Design review of the part shown in the three views and the two pictorial views. Dimensions are in mm from the part's minimum x, y and z. A direction names the side the tool comes from. Give positions to 0.01 mm unless a question says otherwise; leave off trailing zeros. Write each loop counter-clockwise with the first axis right and the second up, starting at its lowest first coordinate (ties: lowest second). Pieces come first, ordered by that corner, then holes. Notation, with made-up numbers: M -38.5,15.25 L 3.5,15.25 A20 cw 3.5,39.25 Z; hole C -20,36.25 d6. An arc over 180 degrees is marked long. Write item = value, one per line.
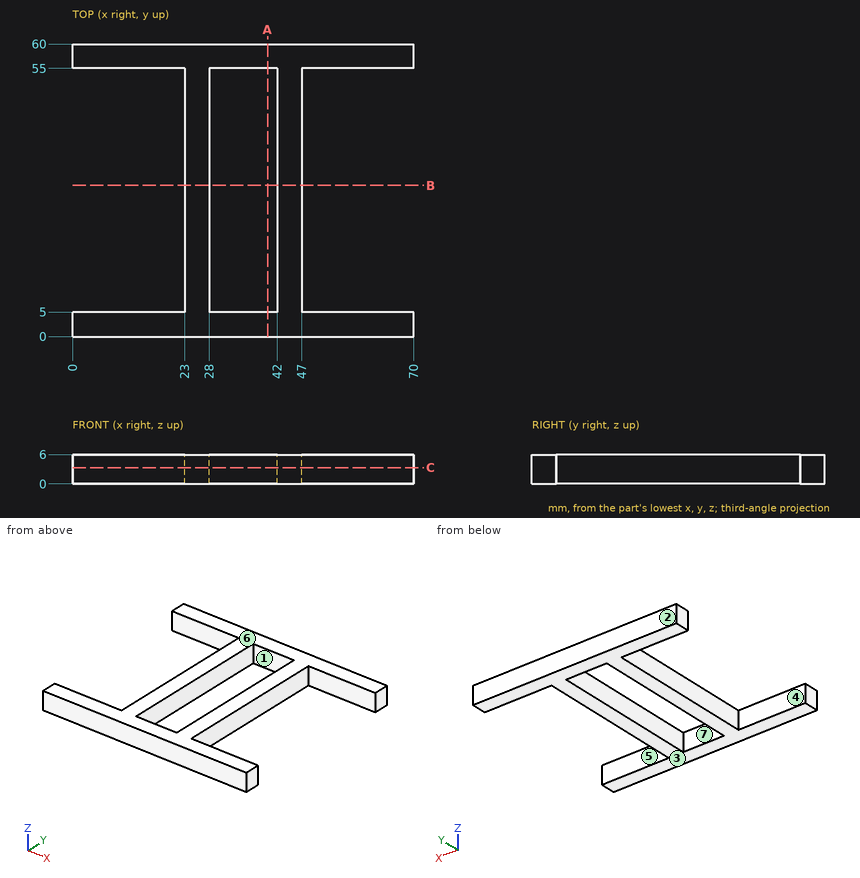
1. We need section A-A, the plane x = 40. Write out the cut boundary in (y, z).
Responses:
outline = M 0,0 L 5,0 L 5,6 L 0,6 Z; M 55,0 L 60,0 L 60,6 L 55,6 Z
2. We need section B-B, the plane y = 31. Write out the cut boundary in (x, z), then the cut area to 3 significant figures.
Responses:
outline = M 23,0 L 28,0 L 28,6 L 23,6 Z; M 42,0 L 47,0 L 47,6 L 42,6 Z
area = 60.0 mm2
3. Machinability: for the marked faces 4, 5, 6 and 7, which of the approach directions +Z, -Z, +X, -X, +Y, -Y give a long, thin tool a straight path to every point of the face, cutting with its end or side? Answer none if there is none.
Responses:
face_4 = +Z, -Z, -X
face_5 = +Z, -Z, +X
face_6 = +Z, +X, -X, +Y, -Y
face_7 = +Z, -Z
4. The part is to be moulded in two halves that separate along Y. For the marked faces 1, 2 and 3, say which applies: +Y half, -Y half, draft (parallel to the pull), parting line (faces both ways), or undercut.
Responses:
face_1 = undercut
face_2 = +Y half
face_3 = draft
5. We need section C-C, the plane z = 3.35. Write out the cut boundary in (x, y), then the cut area to 3 significant figures.
Responses:
outline = M 0,0 L 70,0 L 70,5 L 47,5 L 47,55 L 70,55 L 70,60 L 0,60 L 0,55 L 23,55 L 23,5 L 0,5 Z; hole M 28,5 L 42,5 L 42,55 L 28,55 Z
area = 1,200 mm2
6. For line 1 along Y through (x, z) = (58.5, 1); line 2 along X through (y, z) = (29.5, 0.7), list the stretches that pass through material, from the lowest coordinate up. Write a range as from..to.
Responses:
line_1 = 0..5, 55..60
line_2 = 23..28, 42..47
7. Insertion check: P1, Ø1.5, axis at y = 48.5, z = 2, coming from the +X side; P2, Ø10, axis at x = 56.5, y = 19, coming from the +Z side; P3, Ø1.8, axis at y = 24, z = 3.5, coming from the -X side. Each pin has a flat end and moves straight along its axis. Give the tip position at first contact, or say it passes through.
Responses:
P1 = 47
P2 = through
P3 = 23
